Geometry: final body of the model. Coordinates: model frame, mm. Face numbers are marked on the shaded views. A direction names the side the tool comes from. Give positions to 0.01 mm unless a question says otherwise; leave off trailing zeros. Write each loop counter-clockwise with the first axis right and the second up, starting at its lowest first coordinate (ties: lowest second). Pieces come first, ordered by that corner, then holes. Notation, with made-up numbers: M -11,67 L -6,67 A25 cw -6,82 Z; hole C -18.75,0.5 d5. An arc over 180 degrees is marked long. Use a Markdown table: item, result. Add a question column.
1) Draft query along Z for the marked faces 1, 2, 3 and 4. Return one class per face: +Z half, -Z half, draft (parallel to the pull), parting line (faces both ways), or undercut.
2) Pin query (flat end, axial travel): pin 1 (6 mm diameter, centred on y = 3.5, z = 9, fed in from -X); pin 2 (5 mm diameter, centred on x = -13, z = 7.5, fed in from -Y); pin 3 (1.5 mm diameter, centred on y = 2.5, z = -12.5, fed in from -X). Return the tip coordinate at first contact, or that it passes through.
3) Section D-D on z = 24.5. Return the cut outline in (x, y).
4) Set-up query: the marked faces 5, 6 and 7. Return all of +Z, -Z, +X, -X, +Y, -Y with unobstructed straight access to the full face (end or side cutting, diameter ignored); none if empty.
5) Section A-A on x = -28. Return the cut outline in (y, z).
6) Section B-B on y = 9.5. Return the cut outline in (x, z).
7) Line query: line 1 (X direction, y = 2.75, z = 19); line 2 (Z direction, x = -35, y = 6.5); line 3 (X direction, y = 1, z = -22). Output: solid intervals per line, ascending.
8) Section C-C on y = 2.75. State how many separate pieces and enclosed holes the cut face has, then the cut area to 3 significant figures.
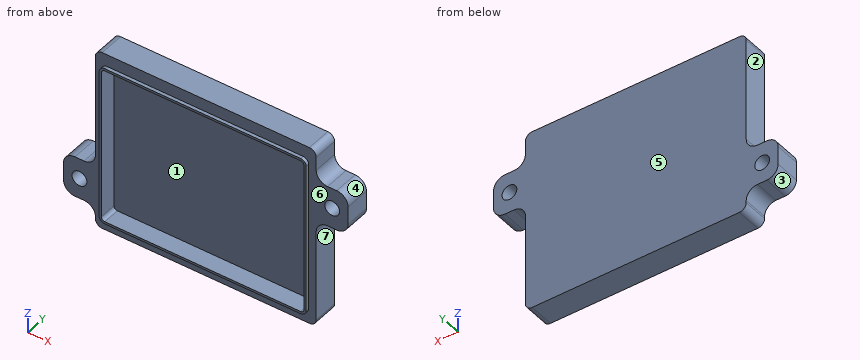
```python
from build123d import *

# Parameters (mm, degrees)
SKETCH1_W           = 97
SKETCH1_H           = 80.401218893
BOSS_EXTRUDE1_DEPTH = 12.6
CUT_EXTRUDE2_START  = -5
CUT_EXTRUDE2_DEPTH  = 10
SKETCH6_W           = 97
SKETCH6_H           = 80.401218893
CUT_EXTRUDE3_DEPTH  = 1.5
FILLET1_R           = 3
SKETCH7_W           = 18
SKETCH7_H           = 11.1
BOSS_EXTRUDE2_DEPTH = 14
SKETCH8_W           = 18
SKETCH8_H           = 11.1
BOSS_EXTRUDE3_DEPTH = 14
FILLET2_R           = 5
SKETCH9_R           = 3.25
CUT_EXTRUDE4_DEPTH  = 13.6


with BuildPart() as part:
    # Sketch1 → Boss-Extrude1 (new body)
    with BuildSketch(Plane(origin=(0, 0, 0), x_dir=(1, 0, 0), z_dir=(0, 1, 0))):
        with Locations((3.433898335, -1.804923378)):
            Rectangle(SKETCH1_W, SKETCH1_H)
    extrude(amount=BOSS_EXTRUDE1_DEPTH)

    # Sketch3 → Cut-Extrude2 (cut)
    with BuildSketch(Plane(origin=(0, 12.6, 0), x_dir=(1, 0, 0), z_dir=(0, 1, 0)).offset(CUT_EXTRUDE2_START)):
        with BuildLine():
            Line((-41.366101665, 31.831649434), (-41.366101665, -34.168350566))
            ThreePointArc((-41.366101665, -34.168350566), (-40.926761836, -35.229010737), (-39.866101665, -35.668350566))
            Line((-39.866101665, -35.668350566), (46.133898335, -35.668350566))
            ThreePointArc((46.133898335, -35.668350566), (47.194558507, -35.229010737), (47.633898335, -34.168350566))
            Line((47.633898335, -34.168350566), (47.633898335, 31.831649434))
            ThreePointArc((47.633898335, 31.831649434), (47.194558507, 32.892309606), (46.133898335, 33.331649434))
            Line((46.133898335, 33.331649434), (-39.866101665, 33.331649434))
            ThreePointArc((-39.866101665, 33.331649434), (-40.926761836, 32.892309606), (-41.366101665, 31.831649434))
        make_face()
    extrude(amount=-CUT_EXTRUDE2_DEPTH, mode=Mode.SUBTRACT)

    # Sketch6 → Cut-Extrude3 (cut)
    with BuildSketch(Plane.XZ):
        with Locations((3.433898335, 1.804923378)):
            Rectangle(SKETCH6_W, SKETCH6_H)
        with BuildLine():
            Line((-39.866101665, -34.331649434), (46.133898335, -34.331649434))
            ThreePointArc((46.133898335, -34.331649434), (47.901665288, -33.599416387), (48.633898335, -31.831649434))
            Line((48.633898335, -31.831649434), (48.633898335, 34.168350566))
            ThreePointArc((48.633898335, 34.168350566), (47.901665288, 35.936117519), (46.133898335, 36.668350566))
            Line((46.133898335, 36.668350566), (-39.866101665, 36.668350566))
            ThreePointArc((-39.866101665, 36.668350566), (-41.633868617, 35.936117519), (-42.366101665, 34.168350566))
            Line((-42.366101665, 34.168350566), (-42.366101665, -31.831649434))
            ThreePointArc((-42.366101665, -31.831649434), (-41.633868617, -33.599416387), (-39.866101665, -34.331649434))
        make_face(mode=Mode.SUBTRACT)
    extrude(amount=-CUT_EXTRUDE3_DEPTH, mode=Mode.SUBTRACT)

    # Fillet1
    fillet1_edges = [part.edges().sort_by_distance(p)[0] for p in [
        (51.933898335, 7.05, 42.005532825),
        (-45.066101665, 7.05, 42.005532825),
        (-45.066101665, 7.05, -38.395686068),
        (51.933898335, 7.05, -38.395686068),
    ]]
    fillet(fillet1_edges, radius=FILLET1_R)

    # Sketch7 → Boss-Extrude2 (add)
    with BuildSketch(Plane.ZY.offset(45.066101665)):
        with Locations((-20.395686068, 7.05)):
            Rectangle(SKETCH7_W, SKETCH7_H)
    extrude(amount=BOSS_EXTRUDE2_DEPTH)

    # Sketch8 → Boss-Extrude3 (add)
    with BuildSketch(Plane(origin=(51.933898335, 0, 0), x_dir=(0, 0, -1), z_dir=(1, 0, 0))):
        with Locations((-19.005532825, 7.05)):
            Rectangle(SKETCH8_W, SKETCH8_H)
    extrude(amount=BOSS_EXTRUDE3_DEPTH)

    # Fillet2
    fillet2_edges = [part.edges().sort_by_distance(p)[0] for p in [
        (-45.066101665, 7.05, -11.395686068),
        (-45.066101665, 7.05, -29.395686068),
        (-59.066101665, 7.05, -11.395686068),
        (-59.066101665, 7.05, -29.395686068),
        (51.933898335, 7.05, 10.005532825),
        (51.933898335, 7.05, 28.005532825),
        (65.933898335, 7.05, 10.005532825),
        (65.933898335, 7.05, 28.005532825),
    ]]
    fillet(fillet2_edges, radius=FILLET2_R)

    # Sketch9 → Cut-Extrude4 (cut, through all)
    with BuildSketch(Plane(origin=(0, 12.6, 0), x_dir=(1, 0, 0), z_dir=(0, 1, 0))):
        with Locations((58.933898335, -19.005532825)):
            Circle(SKETCH9_R)
        with Locations((-52.066101665, 20.395686068)):
            Circle(SKETCH9_R)
    extrude(amount=-CUT_EXTRUDE4_DEPTH, mode=Mode.SUBTRACT)


solid = part.part
```
Found:
| question | item | result |
|---|---|---|
| 1 | face 1 | undercut |
| 1 | face 2 | draft |
| 1 | face 3 | -Z half |
| 1 | face 4 | +Z half |
| 2 | pin 1 | x = -45.07 |
| 2 | pin 2 | y = 7.6 |
| 2 | pin 3 | x = -57.95 |
| 3 | outline | M -45.07,1.5 L -42.37,1.5 L -42.37,0 L -41.37,0 L -41.37,7.6 L 47.63,7.6 L 47.63,0 L 48.63,0 L 48.63,1.5 L 65.71,1.5 L 65.71,12.6 L -45.07,12.6 Z |
| 4 | face 5 | +Z, -Z, +X, -X, +Y |
| 4 | face 6 | -Y |
| 4 | face 7 | -Z, +X, +Y, -Y |
| 5 | outline | M 0,-34.33 L 1.5,-34.33 L 1.5,-38.4 L 12.6,-38.4 L 12.6,42.01 L 1.5,42.01 L 1.5,36.67 L 0,36.67 L 0,35.67 L 7.6,35.67 L 7.6,-33.33 L 0,-33.33 Z |
| 6 | outline | M -59.07,-24.4 A5 ccw -54.07,-29.4 L -50.07,-29.4 A5 cw -45.07,-34.4 L -45.07,-35.4 A3 ccw -42.07,-38.4 L 48.93,-38.4 A3 ccw 51.93,-35.4 L 51.93,5.01 A5 cw 56.93,10.01 L 60.93,10.01 A5 ccw 65.93,15.01 L 65.93,23.01 A5 ccw 60.93,28.01 L 56.93,28.01 A5 cw 51.93,33.01 L 51.93,39.01 A3 ccw 48.93,42.01 L -42.07,42.01 A3 ccw -45.07,39.01 L -45.07,-6.4 A5 cw -50.07,-11.4 L -54.07,-11.4 A5 ccw -59.07,-16.4 Z; hole C -52.07,-20.4 d6.5; hole C 58.93,19.01 d6.5 |
| 7 | line 1 | -45.07 to -41.37, 47.63 to 55.68, 62.18 to 65.93 |
| 7 | line 2 | -38.4 to -33.33, 35.67 to 42.01 |
| 7 | line 3 | -42.37 to -41.37, 47.63 to 48.63 |
| 8 | separate pieces | 1 |
| 8 | enclosed holes | 3 |
| 8 | area | 2,090 mm² |
